Part print with two shaded views. Sizes in mm from the minimum x, y, z corner. A direction names the side the tool comes from. Give positions to 0.01 mm unless a question says otherwise; leave off trailing zeros. Write each loop counter-clockwise with the first axis right and the second up, starting at its lowest first coordinate (ties: lowest second). Pieces come first, ordered by that corner, then holes. Notation, with made-up numbers: M 34.25,70.5 L 65.25,70.5 A22 ccw 65.25,81.5 Z; hole C 66,-19.75 d6. An arc over 180 degrees is marked long. Return JSON: item names as keys, results as strings. Group by question number.
Q1. Band-saw the part on C-C, the plane x = 109.5. Give the cut face in (y, z).
Q2. Band-saw the part on D-D, the plane z = 49. Give the cut face in (x, y), then the cut area to 3 significant figures.
Q3. Tool access for the marked faces 1, 2, 3, 4 and 5: list every direction of +Z, -Z, +X, -X, +Y, -Y with a clear straight run to the whole face (end or side of a thin tool).
Q4. Wall check: probe 1 along X at (y, z) = (52.5, 42.5) (1 decimal); probe 2 along Z at (x, y) = (188.5, 69.5) (1 decimal); probe 3 along Z at (x, y) = (140, 68). Give the ranges that are in metal, low to high.
Q5. Band-saw the part on A-A, the plane z = 22. Give the cut face in (x, y) (1 decimal).
Q6. Flat gauge pins, fed straight in: pin 1 Ø19.5 at (x, y) = (40, 29) entering from -Z (1 decimal); pin 2 Ø8.5 at (y, z) = (47.5, 37) entering from +X (3 decimals); pin 3 Ø6 at (x, y) = (155.5, 59.5) entering from +Z. Where does each tip first touch, or does it go through?
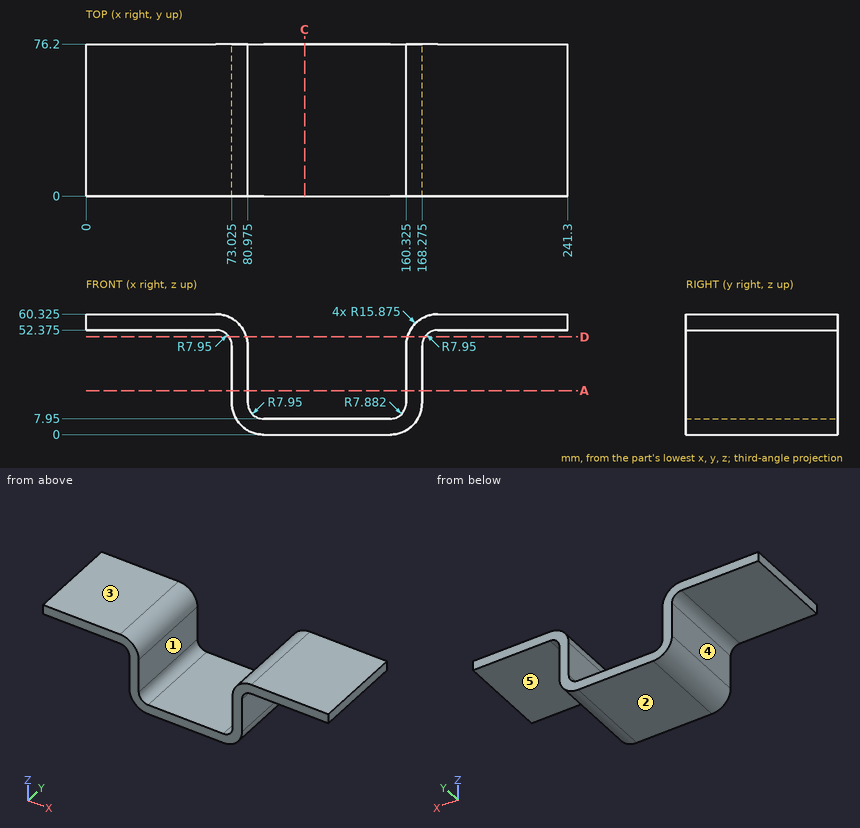
From the geometry:
{
 "1": {"outline": "M 0,0 L 76.2,0 L 76.2,7.95 L 0,7.95 Z"},
 "2": {"outline": "M 71.58,0 L 80.31,0 L 80.31,76.2 L 71.58,76.2 Z; M 160.99,0 L 169.72,0 L 169.72,76.2 L 160.99,76.2 Z", "area": "1,330 mm^2"},
 "3": {"face 1": "+Z, +Y, -Y", "face 2": "-Z, +X, -X, +Y, -Y", "face 3": "+Z, +X, -X, +Y, -Y", "face 4": "-Z, -X, +Y, -Y", "face 5": "-Z, +X, +Y, -Y"},
 "4": {"probe 1": "x = 73 to 81, 160.3 to 168.3", "probe 2": "z = 52.4 to 60.3", "probe 3": "z = 0 to 7.95"},
 "5": {"outline": "M 73,0 L 81,0 L 81,76.2 L 73,76.2 Z; M 160.3,0 L 168.3,0 L 168.3,76.2 L 160.3,76.2 Z"},
 "6": {"pin 1": "stops at z = 52.4", "pin 2": "stops at x = 168.275", "pin 3": "stops at z = 10.79"}
}
